Verification items for the finished model (mm, model axes). A direction names the side the tool comes from. Coordinates: 2 decimals unless noted, no trailing zeros. Order: outer loops, then holes, each group sorted by start corner. A loop starts at its lowest first (then second) coordinate and runs counter-clockwise, first axis right, second up. Notation, with made-up numbers: (-21.5, 37) -> (-2.5, 37) arc R12 ccw to (-2.5, 56) -> close; hole circle Ø10 at (-22.75, 65.5). An arc over 180 degrees is marked (long way). Use CSV: the item, a comma, the result in double quotes. Start each with the question number.
1) Tool access check on faces 4 (the flat face through (4, 0, 0)), 5 (the cylindrical face through (3.174, 0.057, 1.479)), 6 (the flat face through (1.462, -5, 1)). Record the directions out of +Z, -Z, +X, -X, +Y, -Y that give a thin tool (end or side, any length) a straight path to the whole face; none if there is none.
2) Scan lines: line 1 along Y through (x, z) = (0, 2.6) (3 decimals); line 2 along Y through (x, z) = (-2.5, 0.3); line 3 along Y through (x, z) = (-2, 1.15). Record each from-to range of solid material in increasing order.
3) Go/stop test with flat-tipped pins: pin 1 (1 mm diameter, centred on x = -6.5, z = 2, fed in from +Y); pin 2 (1.4 mm diameter, centred on x = 0.5, z = 1.5, fed in from -Y); pin 3 (0.9 mm diameter, centred on y = 3.5, z = 1.5, fed in from +X); pin 4 (5 mm diameter, centred on x = 2, y = 1, fed in from +Z). Record where each tip stops, or that it passes through.
4) Release check for a two-part mould opening along Y. For faces 1 (the flat face through (-1.448, 4, 1)), 2 (the cylindrical face through (-3.175, -0.04, 1.479)), 3 (the cylindrical face through (1.99, -8.45, 1.52)) record: released by +Y, released by -Y, zero draft, split by the parting line, or undercut.
5) Sectioned sample at D-D on x = 0. Record the boundary of the cut face in (y, z) (3 decimals).
6) Sectioned sample at C-C on x = -2. Record the boundary of the cut face in (y, z).
7) Sectioned sample at A-A on y = 0. Record the boundary of the cut face in (x, z) (3 decimals).
from build123d import *

# Parameters (mm, degrees)
EXTRUDE_1_DEPTH = 3
FILLET_1_R      = 1.27


with BuildPart() as part:
    # 스케치1 → 보스-돌출1 (new body)
    with BuildSketch(Plane.XY):
        with BuildLine():
            Line((-1.4475, 5.825839477), (1.4475, 5.825839477))
            Line((1.4475, 5.825839477), (1.4475, 2.825839477))
            ThreePointArc((1.4475, 2.825839477), (3.174988787, 0.008438217), (1.4625, -2.818105525))
            Line((1.4625, -2.818105525), (1.4625, -9.057688378))
            ThreePointArc((1.4625, -9.057688378), (0, 9.175), (-1.4625, -9.057688378))
            Line((-1.4625, -9.057688378), (-1.4625, -2.818105525))
            ThreePointArc((-1.4625, -2.818105525), (-3.174988787, 0.008438217), (-1.4475, 2.825839477))
            Line((-1.4475, 2.825839477), (-1.4475, 5.825839477))
        make_face()
    extrude(amount=EXTRUDE_1_DEPTH)

    # 필렛1
    fillet_1_edges = [part.edges().sort_by_distance(p)[0] for p in [
        (-1.4625, -9.057688378, 1.5),
        (1.4625, -9.057688378, 1.5),
    ]]
    fillet(fillet_1_edges, radius=FILLET_1_R)


solid = part.part
Answers follow:
1,face 4,"-Z, +X, -X, +Y, -Y"
1,face 5,"+Z, -Z"
1,face 6,"+Z, -Z, -Y"
2,line 1,"y = 5.826 to 9.175"
2,line 2,"y = -8.67 to -1.96, 1.96 to 8.83"
2,line 3,"y = -8.46 to -2.47, 2.47 to 8.95"
3,pin 1,"stops at y = 6.94"
3,pin 2,"stops at y = 5.83"
3,pin 3,"stops at x = 8.65"
3,pin 4,"stops at z = 3"
4,face 1,"zero draft"
4,face 2,"undercut"
4,face 3,"released by -Y"
5,outline,"(5.826, 0) -> (9.175, 0) -> (9.175, 3) -> (5.826, 3) -> close"
6,outline,"(-8.46, 0) -> (-2.47, 0) -> (-2.47, 3) -> (-8.46, 3) -> close; (2.47, 0) -> (8.95, 0) -> (8.95, 3) -> (2.47, 3) -> close"
7,outline,"(-9.175, 0) -> (-3.175, 0) -> (-3.175, 3) -> (-9.175, 3) -> close; (3.175, 0) -> (9.175, 0) -> (9.175, 3) -> (3.175, 3) -> close"
